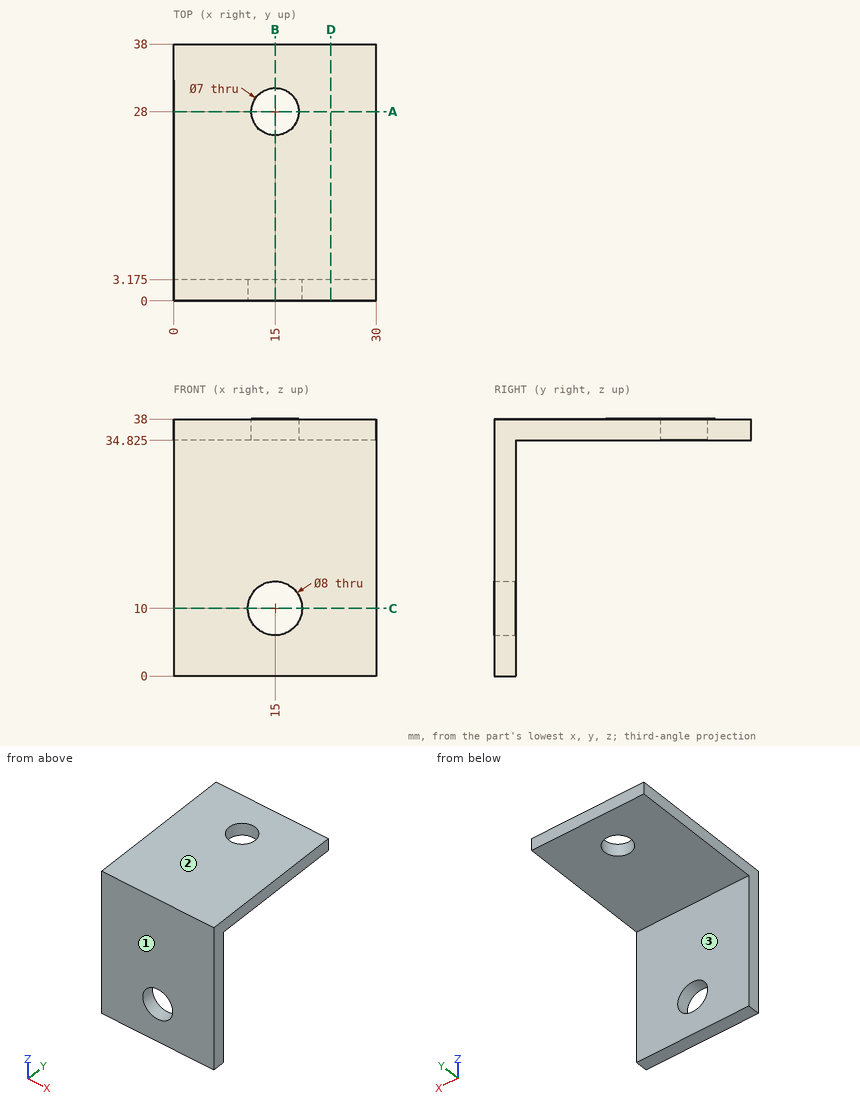
Input: dimensioned drawing with shaded views. Units: mm. Origin: part minimum x, y, z. Give positions to 0.01 mm unless a question says otherwise; leave off trailing zeros. Loops run counter-clockwise (first coordinate to the right, second up) from the corner with the lowest first, then second, coordinate; pieces in that order, holes last. Notation, with made-up numbers: (28.5, 11.25) - (78.5, 11.25) arc R23 ccw to (78.5, 32.25) - close; hole circle Ø2 at (-11.5, 66). An arc over 180 degrees is marked (long way). Answer as CSV lines item,"result". Start each with the question number.
(1) Section query C-C (z = 10). Output: boundary loops of the cut face in (x, y) (3 decimals).
(2) Section query A-A (y = 28). Output: boundary loops of the cut face in (x, z) (3 decimals).
(3) Pin query (flat end, axial travel): P1, Ø13, axis at x = 15, z = 10, coming from the +Y side (3 decimals); P2, Ø15, axis at x = 15, y = 15, coming from the -Z side (3 decimals); P3, Ø5, axis at y = 23, z = 32.5, coming from the +X side. Return the tip coordinate at first contact, or that it passes through.
(4) Section query D-D (x = 23.25). Output: boundary loops of the cut face in (y, z) (3 decimals).
(5) Mould query, pull axis Y, two halves, no side actions, for the marked faces 1, 2 and 3. Classes: +Y half, -Y half, draft (parallel to the pull), parting line (faces both ways), or undercut.
(6) Ray query, line 1 along Z through (x, y) = (15, 1.45); line 2 along Y through (x, z) = (15, 36.5); line 3 along Z through (x, y) = (14.25, 9) (3 decimals). Return the intervals inside material, ascending. Write a range as [from, to].
(7) Section query B-B (x = 15). Output: boundary loops of the cut face in (y, z) (3 decimals), and give its area (3 significant figures).
Worked answers:
1,outline,"(0, 0) - (11, 0) - (11, 3.175) - (0, 3.175) - close; (19, 0) - (30, 0) - (30, 3.175) - (19, 3.175) - close"
2,outline,"(0, 34.825) - (11.5, 34.825) - (11.5, 38) - (0, 38) - close; (18.5, 34.825) - (30, 34.825) - (30, 38) - (18.5, 38) - close"
3,P1,"stops at y = 3.175"
3,P2,"stops at z = 34.825"
3,P3,"stops at x = 30"
4,outline,"(0, 0) - (3.175, 0) - (3.175, 34.825) - (38, 34.825) - (38, 38) - (0, 38) - close"
5,face 1,"-Y half"
5,face 2,"draft"
5,face 3,"+Y half"
6,line 1,"z = [0, 6], [14, 38]"
6,line 2,"y = [0, 24.5], [31.5, 38]"
6,line 3,"z = [34.825, 38]"
7,outline,"(0, 0) - (3.175, 0) - (3.175, 6) - (0, 6) - close; (0, 14) - (3.175, 14) - (3.175, 34.825) - (24.5, 34.825) - (24.5, 38) - (0, 38) - close; (31.5, 34.825) - (38, 34.825) - (38, 38) - (31.5, 38) - close"
7,area,"184 mm^2"
